Verification items for the finished model (mm, model axes). A direction names the side the tool comes from. Give positions to 0.01 mm unless a question says otherwise; leave off trailing zeros. Order: outer loops, then holes, each group sorted by start corner. A loop starts at its lowest first (then second) coordinate and runs counter-clockwise, first axis right, second up. Notation, with made-up numbers: (57.25, -16) -> (68.25, -16) arc R25 ccw to (68.25, 10) -> close; hole circle Ø10 at (-27.75, 72.5). An arc over 180 degrees is marked (long way). One line per question, with ' | ' between items. Start each with the question number.
Q1. Section check C-C on x = 10. Record the cut outline in (y, z) (3 decimals).
Q2. Section check D-D on z = -8.5. Record the cut outline in (x, y) (3 decimals).
Q3. Section check B-B on y = 6. Record the cut outline in (x, z) (3 decimals), plus the area to 3 significant figures.
Q4. Material ranges on probe 1 along Z at (x, y) = (10, 3) (3 decimals); probe 2 along Y at (x, z) = (16, -29) (3 decimals); probe 3 along X at (y, z) = (-14, -38), recorded low to high. Write a range as [from, to].
Q5. Section check A-A on x = 0. Record the cut outline in (y, z) (3 decimals), plus the area to 3 significant figures.
Q6. Access from +Z, -Z, +X, -X, +Y, -Y to the whole of each face (thin tool, end or side, straight path). Record for faces 4 (the flat face through (0.2, 2.6, 0)), 5 (the flat face through (25, -14, -13.335)), 6 (the flat face through (40.259, -14, -29)).
Q7. Mould release check, pull along X, two halves, no side actions. Record for faces 1 (the flat face through (24.862, -14, -40)), 2 (the flat face through (7, -14, -34.925)), 3 (the cylindrical face through (-0.569, 11.634, 1.565)): released by +X, released by -X, zero draft, split by the parting line, or undercut.
Q8. Go/stop test with flat-tipped pins: pin 1 (1.6 mm diameter, centred on x = 22, y = -13.5, fed in from +Z) (3 decimals); pin 2 (8.5 mm diameter, centred on y = 5.5, z = -3, fed in from +X) (3 decimals); pin 3 (5 mm diameter, centred on x = 7.5, z = -31, fed in from +Y) (3 decimals). Record where each tip stops, or that it passes through.
from build123d import *

# Parameters (mm, degrees)
SKETCH1_R                    = 4.3688
BOSS_EXTRUDE1_DEPTH          = 3.175
EDGE_FLANGE1_STRIP_W         = 15.900000204
EDGE_FLANGE1_STRIP_H         = 3.175
EDGE_FLANGE1_STRIP_CUT_DEPTH = 21.59
EDGE_FLANGE1_DEPTH           = 21.59
EDGE_FLANGE1_FLAT_DEPTH      = 3.175


# Sheet-metal steps are written as plain solids
with BuildPart() as part:
    # Sketch1 → Boss-Extrude1 (new body)
    with BuildSketch(Plane.XY):
        Polygon((-10.795, 15.24), (10.795, 15.24), (10.795, -15.24), (-10.795, -15.24), (-10.795, -1.27), align=None)
        with Locations((0, 7.3025)):
            Circle(SKETCH1_R, mode=Mode.SUBTRACT)
    extrude(amount=BOSS_EXTRUDE1_DEPTH)

    # Edge-Flange1 strip (across the edge) → Edge-Flange1 strip cut (cut)
    with BuildSketch(Plane(origin=(10.795, -15.24, 0), x_dir=(0, 1, 0), z_dir=(-1, 0, 0))):
        with Locations((-3.175, -1.5875)):
            Rectangle(EDGE_FLANGE1_STRIP_W, EDGE_FLANGE1_STRIP_H)
    extrude(amount=EDGE_FLANGE1_STRIP_CUT_DEPTH, mode=Mode.SUBTRACT)

    # Edge-Flange1 bend section (across the edge) → Edge-Flange1 (add)
    with BuildSketch(Plane(origin=(10.795, -15.24, 0), x_dir=(0, 1, 0), z_dir=(-1, 0, 0))):
        with BuildLine():
            Line((0, 1.600000102), (3.175, 1.600000102))
            ThreePointArc((3.175, 1.600000102), (3.64362918, 0.46862918), (4.775000102, 0))
            Line((4.775000102, 0), (4.775000102, -3.175))
            ThreePointArc((4.775000102, -3.175), (1.39856515, -1.77643485), (0, 1.600000102))
        make_face()
    extrude(amount=EDGE_FLANGE1_DEPTH)

    # Edge-Flange1 profile (on flange) → Edge-Flange1 flat (add)
    with BuildSketch(Plane(origin=(0, -15.24, 0), x_dir=(1, 0, 0), z_dir=(0, 1, 0))):
        Polygon((-10.795, 1.600000102), (10.795, 1.600000102), (10.795, 13.335), (33.655, 13.335), (38.735, 13.335), (40.259, 13.335), (40.259, 45.085), (38.735, 45.085), (26.386399264, 45.085), (24.862399264, 45.085), (24.862399264, 34.925), (21.306399264, 34.925), (16.226399264, 34.925), (10.795, 34.925), (-10.795, 34.925), (-10.795, 13.335), align=None)
    extrude(amount=EDGE_FLANGE1_FLAT_DEPTH)


solid = part.part
Filled in:
1) outline: (-15.24, -34.925) -> (-12.065, -34.925) -> (-12.065, -1.6) arc R1.6 cw to (-10.465, 0) -> (15.24, 0) -> (15.24, 3.175) -> (-10.465, 3.175) arc R4.775 ccw to (-15.24, -1.6) -> close
2) outline: (-10.795, -15.24) -> (10.795, -15.24) -> (10.795, -12.065) -> (-10.795, -12.065) -> close
3) outline: (-10.795, 0) -> (-4.17, 0) -> (-4.17, 3.175) -> (-10.795, 3.175) -> close; (4.17, 0) -> (10.795, 0) -> (10.795, 3.175) -> (4.17, 3.175) -> close | area: 42.1 mm²
4) probe 1: [0, 3.175] | probe 2: [-15.24, -12.065] | probe 3: [24.86, 40.26]
5) outline: (-15.24, -34.925) -> (-12.065, -34.925) -> (-12.065, -1.6) arc R1.6 cw to (-10.465, 0) -> (2.934, 0) -> (2.934, 3.175) -> (-10.465, 3.175) arc R4.775 ccw to (-15.24, -1.6) -> close; (11.671, 0) -> (15.24, 0) -> (15.24, 3.175) -> (11.671, 3.175) -> close | area: 176 mm²
6) face 4: -Z, +X, -X, +Y | face 5: +Z, +X, +Y, -Y | face 6: +Z, -Z, +X, +Y, -Y
7) face 1: released by -X | face 2: zero draft | face 3: undercut
8) pin 1: z = -13.335 | pin 2: x = 10.795 | pin 3: y = -12.065
